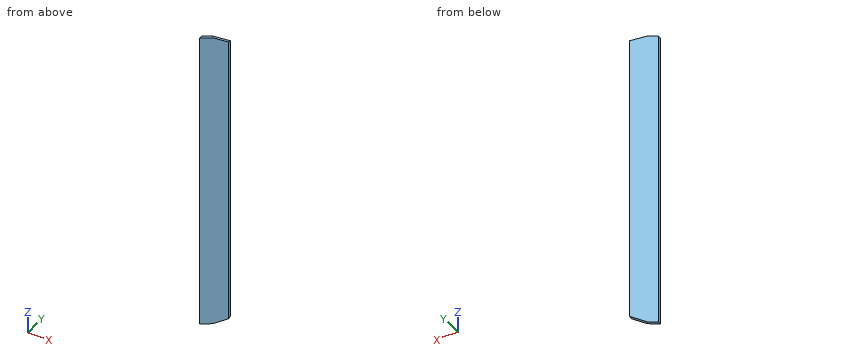
from build123d import *

# Parameters (mm, degrees)
SALIENTE_EXTRUIR2_DEPTH      = 21
SALIENTE_EXTRUIR2_DEPTH_BACK = 77
CORTAR_EXTRUIR2_DEPTH        = 5.534624471


with BuildPart() as part:
    # Croquis1 → Saliente-Extruir2 (new body, two sides)
    with BuildSketch(Plane.XY) as saliente_extruir2_sk:
        Polygon((4, -95.47461527), (-2.5, -100), (-2.5, -99), (4, -94.47461527), align=None)
    extrude(amount=SALIENTE_EXTRUIR2_DEPTH)
    extrude(saliente_extruir2_sk.sketch, amount=-SALIENTE_EXTRUIR2_DEPTH_BACK)

    # Croquis3 → Cortar-Extruir2 (cut, through all)
    with BuildSketch(Plane(origin=(45.607014753, -65.507269237, 0), x_dir=(0.820689363, 0.571374632, 0), z_dir=(-0.571374632, 0.820689363, 0))):
        Polygon((-50.697641098, 77), (-50.697641098, 75.231357415), (-55.571592416, 77), align=None)
        Polygon((-50.697641098, -21), (-50.697641098, -19.231357415), (-55.571592416, -21), align=None)
    extrude(amount=-CORTAR_EXTRUIR2_DEPTH, mode=Mode.SUBTRACT)


solid = part.part
Input: part model. Units: mm. Frame: model coordinates. Give positions to 0.01 mm unless a question says otherwise; leave off trailing zeros. Loops run counter-clockwise (first coordinate to the right, second up) from the corner with the lowest first, then second, coordinate; pieces in that order, holes last. Notation, with made-up numbers: (48.25, 41.25) -> (52.25, 41.25) arc R17 cw to (52.25, 66.25) -> close; hole circle Ø1 at (49, 45.5). An arc over 180 degrees is marked (long way). Answer as a JSON object with one key per item and string values. Group by question number.
Item 1: Cut plane A-A, the plane z = -4. Return the cut outline in (x, y), and give its area (3 significant figures).
Item 2: Cut plane B-B, the plane x = 2.5. Return the cut outline in (y, z).
Item 3: Line query: probe 1 along X at (y, z) = (-97.9, -57.5); probe 2 along X at (y, z) = (-94.8, -3); probe 3 along Y at (x, z) = (-2, -13.5). Output: solid intervals per line, ascending.
Item 4: Pin query (flat end, axial travel): P1, Ø2, axis at y = -97, z = -40, coming from the -X side; P2, Ø1, axis at x = -1, z = -41.5, coming from the +Y side. Return the tip coordinate at first contact, or that it passes through.
Checks:
{
 "1": {"outline": "(-2.5, -100) -> (4, -95.47) -> (4, -94.47) -> (-2.5, -99) -> close", "area": "6.50 mm²"},
 "2": {"outline": "(-96.52, -76.1) -> (-95.52, -75.89) -> (-95.52, 19.89) -> (-96.52, 20.1) -> close"},
 "3": {"probe 1": "x = -0.92 to 0.52", "probe 2": "x = 3.53 to 4", "probe 3": "y = -99.65 to -98.65"},
 "4": {"P1": "stops at x = -1.06", "P2": "stops at y = -97.61"}
}
